Input: part model. Units: mm. Frame: model coordinates. A direction names the side the tool comes from. Coordinates: 2 decimals unless noted, no trailing zeros. Loops run counter-clockwise (first coordinate to the right, second up) from the corner with the lowest first, then second, coordinate; pieces in that order, holes last.
```python
from build123d import *

# Parameters (mm, degrees)
CYLINDER_R        = 3.8
CYLINDER_DEPTH    = 50
CYLINDER001_R     = 10
CYLINDER001_DEPTH = 15
BOX001_W          = 12
BOX001_H          = 12
BOX001_DEPTH      = 10
BOX003_W          = 80
BOX003_H          = 4
BOX003_DEPTH      = 10
BOX004_W          = 4
BOX004_H          = 40
BOX004_DEPTH      = 10
CYLINDER003_R     = 2
CYLINDER003_DEPTH = 17
ARRAY001_X_COUNT  = 2
ARRAY001_X_PITCH  = 57
ARRAY001_Y_COUNT  = 2
ARRAY001_Y_PITCH  = 55
BOX002_W          = 61
BOX002_H          = 59
BOX002_DEPTH      = 17
BOX_W             = 65
BOX_H             = 63
BOX_DEPTH         = 17
FILLET_R          = 4
CYLINDER002_R     = 4
CYLINDER002_DEPTH = 17
ARRAY_X_COUNT     = 2
ARRAY_X_PITCH     = 57
ARRAY_Y_COUNT     = 2
ARRAY_Y_PITCH     = 55


with BuildPart() as encoder_hole:
    # Cylinder → Cylinder (new body)
    with BuildSketch(Plane.XY):
        Circle(CYLINDER_R)
    extrude(amount=CYLINDER_DEPTH)


with BuildPart() as encoder_cap:
    # Cylinder001 → Cylinder001 (new body)
    with BuildSketch(Plane.XY.offset(35)):
        Circle(CYLINDER001_R)
    extrude(amount=CYLINDER001_DEPTH)


with BuildPart() as encoder_fusion:
    # Box001 → Box001 (new body)
    with BuildSketch(Plane(origin=(-6, -6, 0), x_dir=(1, 0, 0), z_dir=(0, 0, 1))):
        with Locations((6, 6)):
            Rectangle(BOX001_W, BOX001_H)
    extrude(amount=BOX001_DEPTH)

    # Fusion: union encoder hole, encoder cap
    add(encoder_hole.part)
    add(encoder_cap.part)


with BuildPart() as encoder_fusion_1:
    # Fusion placement: moved
    add(encoder_fusion.part.moved(Location((0, 0, -20))))


with BuildPart() as encoder_clone001:
    # Body001 base: copy of encoder fusion
    add(encoder_fusion_1.part)


with BuildPart() as encoder_clone001_1:
    # Clone001 placement: moved
    add(encoder_clone001.part.moved(Location((0, 0, 20))))


with BuildPart() as encoder_clone001_2:
    # Body001 placement: moved
    add(encoder_clone001_1.part.moved(Location((22, 0, -20))))


with BuildPart() as encoder_compound_clone:
    # Body base: copy of encoder fusion
    add(encoder_fusion_1.part)


with BuildPart() as encoder_compound_clone_1:
    # Clone placement: moved
    add(encoder_compound_clone.part.moved(Location((0, 0, 20))))


with BuildPart() as encoder_compound_clone_2:
    # Body placement: moved
    add(encoder_compound_clone_1.part.moved(Location((44, 0, -20))))

    # Compound: union encoder clone001, encoder fusion
    add(encoder_clone001_2.part)
    add(encoder_fusion_1.part)


with BuildPart() as cube003:
    # Box003 → Box003 (new body)
    with BuildSketch(Plane(origin=(-20, 20, -22), x_dir=(1, 0, 0), z_dir=(0, 0, 1))):
        with Locations((40, 2)):
            Rectangle(BOX003_W, BOX003_H)
    extrude(amount=BOX003_DEPTH)


with BuildPart() as cube004:
    # Box004 → Box004 (new body)
    with BuildSketch(Plane(origin=(14, -40, -22), x_dir=(1, 0, 0), z_dir=(0, 0, 1))):
        with Locations((2, 20)):
            Rectangle(BOX004_W, BOX004_H)
    extrude(amount=BOX004_DEPTH)


with BuildPart() as encoder_box_extract:
    # Cylinder003 → Cylinder003 (new body)
    with BuildSketch(Plane(origin=(-11, -15, -20), x_dir=(1, 0, 0), z_dir=(0, 0, 1))):
        Circle(CYLINDER003_R)
    extrude(amount=CYLINDER003_DEPTH)

    # Array001 X: encoder box extract ×2


with BuildPart() as encoder_box_extract_1:
    add(encoder_box_extract.part)
    with Locations(*[(i * ARRAY001_X_PITCH, 0, 0) for i in range(1, ARRAY001_X_COUNT)]):
        add(encoder_box_extract.part)

    # Array001 Y: encoder box extract ×2


with BuildPart() as encoder_box_extract_2:
    add(encoder_box_extract_1.part)
    with Locations(*[(0, i * ARRAY001_Y_PITCH, 0) for i in range(1, ARRAY001_Y_COUNT)]):
        add(encoder_box_extract_1.part)

    # Fusion002: union encoder compound clone, Cube003, Cube004
    add(encoder_compound_clone_2.part)
    add(cube003.part)
    add(cube004.part)


with BuildPart() as cube002:
    # Box002 → Box002 (new body)
    with BuildSketch(Plane(origin=(-13, -17, -20), x_dir=(1, 0, 0), z_dir=(0, 0, 1))):
        with Locations((30.5, 29.5)):
            Rectangle(BOX002_W, BOX002_H)
    extrude(amount=BOX002_DEPTH)


with BuildPart() as fillet_body:
    # Box → Box (new body)
    with BuildSketch(Plane(origin=(-15, -19, -17), x_dir=(1, 0, 0), z_dir=(0, 0, 1))):
        with Locations((32.5, 31.5)):
            Rectangle(BOX_W, BOX_H)
    extrude(amount=BOX_DEPTH)

    # Cut001: cut Cube002
    add(cube002.part, mode=Mode.SUBTRACT)

    # Fillet
    fillet_edges = [fillet_body.edges().sort_by_distance(p)[0] for p in [
        (-15, -19, -8.5),
        (-15, 44, -8.5),
        (50, -19, -8.5),
        (50, 44, -8.5),
    ]]
    fillet(fillet_edges, radius=FILLET_R)


with BuildPart() as encoder_box_cut:
    # Cylinder002 → Cylinder002 (new body)
    with BuildSketch(Plane(origin=(-11, -15, -17), x_dir=(1, 0, 0), z_dir=(0, 0, 1))):
        Circle(CYLINDER002_R)
    extrude(amount=CYLINDER002_DEPTH)

    # Array X: encoder box cut ×2


with BuildPart() as encoder_box_cut_1:
    add(encoder_box_cut.part)
    with Locations(*[(i * ARRAY_X_PITCH, 0, 0) for i in range(1, ARRAY_X_COUNT)]):
        add(encoder_box_cut.part)

    # Array Y: encoder box cut ×2


with BuildPart() as encoder_box_cut_2:
    add(encoder_box_cut_1.part)
    with Locations(*[(0, i * ARRAY_Y_PITCH, 0) for i in range(1, ARRAY_Y_COUNT)]):
        add(encoder_box_cut_1.part)

    # Fusion001: union Fillet body
    add(fillet_body.part)

    # Cut: cut encoder box extract
    add(encoder_box_extract_2.part, mode=Mode.SUBTRACT)


solid = encoder_box_cut_2.part
```
Item 1: Section query D-D (y = -1). Output: boundary loops of the cut face in (x, z), then the cut area to 3 significant figures.
Result:
outline: (-15, -17) - (-13, -17) - (-13, -3) - (-3.67, -3) - (-3.67, 0) - (-15, 0) - close; (3.67, -3) - (18.33, -3) - (18.33, 0) - (3.67, 0) - close; (25.67, -3) - (40.33, -3) - (40.33, 0) - (25.67, 0) - close; (47.67, -3) - (48, -3) - (48, -10) - (50, -10) - (50, 0) - (47.67, 0) - close
area: 171 mm2
Item 2: Reachability of faces 4 (the face through (46, -13, -10)), 5 (the face through (16, -18, -12)), 6 (the face through (49, 22, -12)) from +Z, -Z, +X, -X, +Y, -Y: full face, straight path, thin tool, end or side. Return the list, or none.
Result:
face 4: -Z
face 5: -Z, -Y
face 6: -Z, +X, -X
Item 3: Mould query, pull axis X, two halves, no side actions, for faces 1 (the face through (-8.12, -12.224, -10.098)), 2 (the face through (-15, 12, -9)), 3 (the face through (49, 13, -17)). Classes: +X half, -X half, draft (parallel to the pull), parting line (faces both ways), or undercut.
Result:
face 1: undercut
face 2: -X half
face 3: draft
Item 4: Line query: L1, parallel to X at y = 0, z = -2.3; L2, parallel to X at y = -9, z = -5.75; L3, parallel to Y at x = 19.5, z = -9. Output: solid intervals per line, ascending.
Result:
L1: x = -15 to -3.8, 3.8 to 18.2, 25.8 to 40.2, 47.8 to 50
L2: x = -15 to -13, 48 to 50
L3: y = -19 to -17, 42 to 44
Item 5: Section query C-C (x = 15). Output: boundary loops of the cut face in (y, z).
Result:
outline: (-19, -12) - (-17, -12) - (-17, -3) - (42, -3) - (42, -17) - (44, -17) - (44, 0) - (-19, 0) - close
Item 6: Section query A-A (x = 0). Output: boundary loops of the cut face in (y, z).
Result:
outline: (-19, -17) - (-17, -17) - (-17, -3) - (-3.8, -3) - (-3.8, 0) - (-19, 0) - close; (3.8, -3) - (42, -3) - (42, -17) - (44, -17) - (44, 0) - (3.8, 0) - close
Item 7: Section query B-B (z = -4). Output: boundary loops of the cut face in (x, y).
Result:
outline: (-15, -15) arc R4 ccw to (-11, -19) - (46, -19) arc R4 ccw to (50, -15) - (50, 40) arc R4 ccw to (46, 44) - (-11, 44) arc R4 ccw to (-15, 40) - close; hole circle Ø4 at (-11, -15); hole (-13, -11.54) arc R4 cw to (-7.54, -17) - (42.54, -17) arc R4 cw to (48, -11.54) - (48, 36.54) arc R4 cw to (42.54, 42) - (-7.54, 42) arc R4 cw to (-13, 36.54) - close; hole circle Ø4 at (-11, 40); hole circle Ø4 at (46, -15); hole circle Ø4 at (46, 40)
Item 8: Contact query for flat-ended pins moving along their axis: P1, Ø0.6, axis at x = 16, y = -17.5, coming from the -Z side; P2, Ø6, axis at x = -5.5, y = 23, coming from the -Z side; P3, Ø1.6, axis at x = 49, z = -13, coming from the -Y side. Output: stop coordinate, or through.
Result:
P1: stops at z = -12
P2: stops at z = -3
P3: stops at y = -18.34
